Geometry: see drawing. Coordinates: mm, zero at the bounding-box minimum. A direction names the side the tool comes from. Round coordinates to 2 decimals unless told otherwise and drop trailing zeros. Loops run counter-clockwise (first coordinate to the right, second up) from the corner with the lowest first, then second, coordinate; pieces in that order, holes last.
(1) First-contact query: pin 1 Ø3 at (y, z) = (13.5, 8.5) entering from -X (1 decimal); pin 2 Ø1 at (y, z) = (7, 7.5) entering from +X (1 decimal); pin 3 Ø5 at (x, y) = (5.5, 14.5) entering from +Z; pin 4 Ø2.5 at (y, z) = (12, 5) entering from -X. Flat tips, straight axial feed; report the tip coordinate or a pass-through.
(2) Section C-C, the plane z = 17. Return the cut outline in (x, y).
(3) Material intervals for probe 1 along Y at (x, z) = (14, 5); probe 2 along Z at (x, y) = (7.5, 9.25); probe 3 along X at (y, z) = (15.5, 2) (1 decimal), sorted ascending.
(4) Section B-B, the plane y = 8.75. Return the cut outline in (x, z) (1 decimal).
(5) Section D-D, the plane z = 2.5. Return the cut outline in (x, y) (1 decimal), plus the area to 3 significant figures.
(6) Set-up query: the marked faces 1, 2 and 3. Return all of +Z, -Z, +X, -X, +Y, -Y with unobstructed straight access to the full face (end or side cutting, diameter ignored); none if empty.
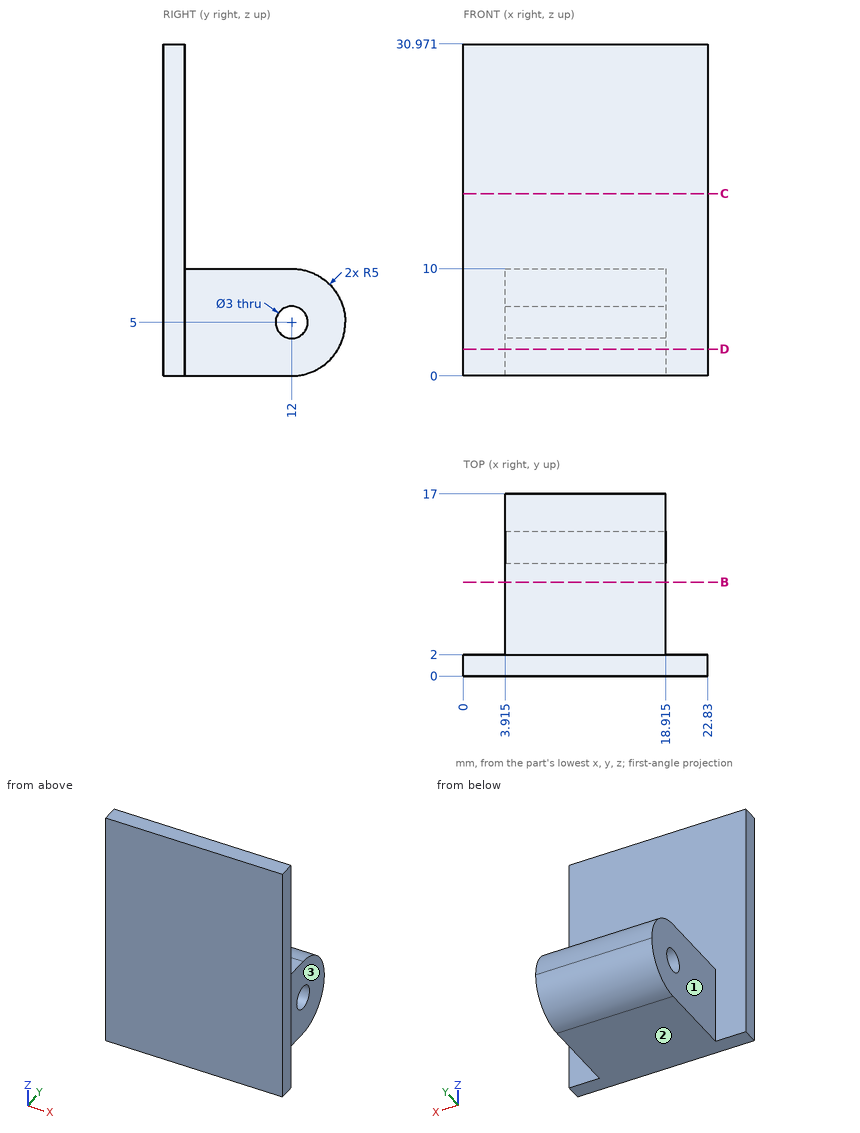
Output values:
1. pin 1: stops at x = 3.9
1. pin 2: stops at x = 18.9
1. pin 3: stops at z = 10
1. pin 4: passes through
2. outline: (0, 0) - (22.83, 0) - (22.83, 2) - (0, 2) - close
3. probe 1: y = 0 to 10.5, 13.5 to 17
3. probe 2: z = 0 to 10
3. probe 3: x = 3.9 to 18.9
4. outline: (3.9, 0) - (18.9, 0) - (18.9, 10) - (3.9, 10) - close
5. outline: (0, 0) - (22.8, 0) - (22.8, 2) - (18.9, 2) - (18.9, 16.3) - (3.9, 16.3) - (3.9, 2) - (0, 2) - close
5. area: 261 mm2
6. face 1: +Z, -Z, -X, +Y
6. face 2: -Z, +X, -X, +Y, -Y
6. face 3: +Z, -Z, +X, +Y
